```python
from build123d import *

# Parameters (mm, degrees)
SKETCH1_W           = 22.225
SKETCH1_H           = 9.525
BOSS_EXTRUDE1_DEPTH = 2.38125
CUT_EXTRUDE1_DEPTH  = 3.38125


with BuildPart() as part:
    # Sketch1 → Boss-Extrude1 (new body)
    with BuildSketch(Plane(origin=(0, 0, 0), x_dir=(1, 0, 0), z_dir=(0, 1, 0))):
        with Locations((11.1125, 4.7625)):
            Rectangle(SKETCH1_W, SKETCH1_H)
    extrude(amount=BOSS_EXTRUDE1_DEPTH)

    # Sketch2 → Cut-Extrude1 (cut, through all)
    with BuildSketch(Plane(origin=(0, 2.38125, 0), x_dir=(1, 0, 0), z_dir=(0, 1, 0))):
        with BuildLine():
            Line((0, 3.175), (4.7625, 3.175))
            ThreePointArc((4.7625, 3.175), (6.35, 4.7625), (4.7625, 6.35))
            Line((4.7625, 6.35), (0, 6.35))
            Line((0, 6.35), (0, 3.175))
        make_face()
        with BuildLine():
            Line((22.225, 6.35), (22.225, 3.175))
            Line((22.225, 3.175), (17.4625, 3.175))
            ThreePointArc((17.4625, 3.175), (15.875, 4.7625), (17.4625, 6.35))
            Line((17.4625, 6.35), (22.225, 6.35))
        make_face()
    extrude(amount=-CUT_EXTRUDE1_DEPTH, mode=Mode.SUBTRACT)


solid = part.part
```
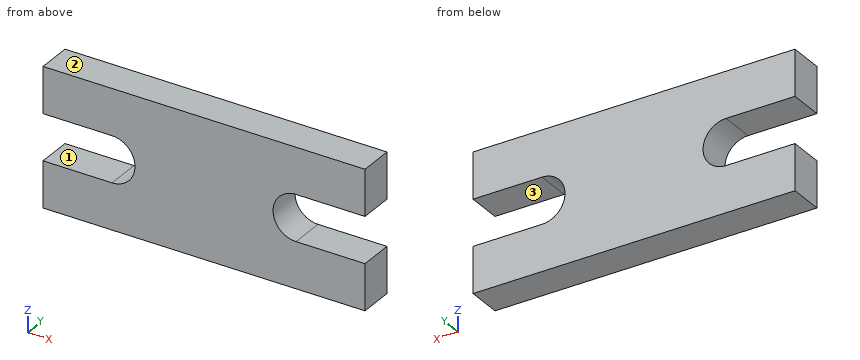
Could you check a few things on this model? Use its own coordinates, in mm. Face numbers are marked on the shaded views. A direction names the side the tool comes from. Round coordinates to 2 decimals unless told otherwise and drop trailing zeros. Order: outer loops, then holes, each group sorted by start corner. A loop starts at its lowest first (then second) coordinate and runs counter-clockwise, first axis right, second up. Notation, with made-up numbers: M -2,10.25 L 33,10.25 A14 ccw 33,19.25 Z; hole C 35.5,23 d5. An arc over 180 degrees is marked long. One line per question, with ' | ' between items. Start each with the question number.
(1) For the marked faces 1, 2 and 3, which set-ups out of +Z, -Z, +X, -X, +Y, -Y let a thin tool reach every point of the face, with its end or its side?
(2) For P1, Ø1.2, axis at x = 3, y = 1.5, coming from the +Z side, with a flat end and sliding along its axis, tell me the tip position at first contact or that it passes through.
(3) Suppose I cut it at A-A on x = 2.25. List the corners of the cut face in (y, z) for me (3 decimals), then the cut area to 3 significant figures.
(4) Suppose I cut it at C-C on x = 16.25. List the corners of the cut face in (y, z) for me (3 decimals), then the cut area to 3 significant figures.
(5) Suppose I cut it at D-D on z = -5.75. List the corners of the cut face in (x, y) for me, then the cut area to 3 significant figures.
(6) Please list where these lines run through material, in increasing order: line 1 along Z through (x, y) = (1, 1.4) (3 decimals); line 2 along Z through (x, y) = (16.5, 1.85) (3 decimals); line 3 along X through (y, z) = (0.55, -5.5).
Geometry results:
1) face 1: -X, +Y, -Y | face 2: +Z, +X, -X, +Y, -Y | face 3: +X, +Y, -Y
2) P1: z = 0
3) outline: M 0,-9.525 L 2.381,-9.525 L 2.381,-6.35 L 0,-6.35 Z; M 0,-3.175 L 2.381,-3.175 L 2.381,0 L 0,0 Z | area: 15.1 mm²
4) outline: M 0,-9.525 L 2.381,-9.525 L 2.381,-5.787 L 0,-5.787 Z; M 0,-3.738 L 2.381,-3.738 L 2.381,0 L 0,0 Z | area: 17.8 mm²
5) outline: M 6.01,0 L 16.22,0 L 16.22,2.38 L 6.01,2.38 Z | area: 24.3 mm²
6) line 1: -9.525 to -6.35, -3.175 to 0 | line 2: -9.525 to -6.025, -3.5 to 0 | line 3: 6.17 to 16.06
